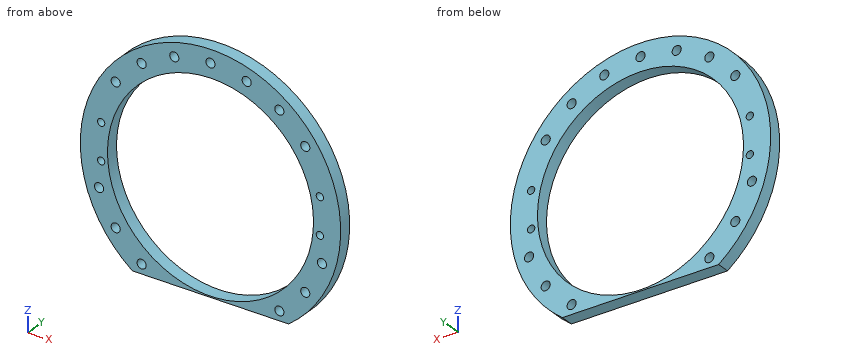
from build123d import *

# Parameters (mm, degrees)
SKETCH4_R           = 50
SKETCH4_R_2         = 39.565
SKETCH4_R_3         = 1.4
SKETCH4_R_4         = 1.75
BOSS_EXTRUDE3_DEPTH = 5
CUT_EXTRUDE1_START  = -40
SKETCH10_W          = 119.00246232
SKETCH10_H          = 31.760523389
CUT_EXTRUDE1_DEPTH  = 31.887234394


with BuildPart() as part:
    # Sketch4 → Boss-Extrude3 (new body)
    with BuildSketch(Plane(origin=(0, 0, 0), x_dir=(1, 0, 0), z_dir=(0, 1, 0))):
        with Locations(Location((0, 0, 0), (0, 0, 270))):
            Circle(SKETCH4_R)
        with Locations(Location((0, 0, 0), (0, 0, 270))):
            Circle(SKETCH4_R_2, mode=Mode.SUBTRACT)
        with Locations(Location((42, -10, 0), (0, 0, 270))):
            Circle(SKETCH4_R_3, mode=Mode.SUBTRACT)
        with Locations(Location((42, 4, 0), (0, 0, 270))):
            Circle(SKETCH4_R_3, mode=Mode.SUBTRACT)
        with Locations(Location((-42, -10, 0), (0, 0, 270))):
            Circle(SKETCH4_R_3, mode=Mode.SUBTRACT)
        with Locations(Location((-42, 4, 0), (0, 0, 270))):
            Circle(SKETCH4_R_3, mode=Mode.SUBTRACT)
        with Locations(Location((0, -45, 0), (0, 0, 270))):
            Circle(SKETCH4_R_4, mode=Mode.SUBTRACT)
        with Locations(Location((-13.905764747, -42.797543233, 0), (0, 0, 270))):
            Circle(SKETCH4_R_4, mode=Mode.SUBTRACT)
        with Locations(Location((-26.450336353, -36.405764747, 0), (0, 0, 270))):
            Circle(SKETCH4_R_4, mode=Mode.SUBTRACT)
        with Locations(Location((-36.405764747, -26.450336353, 0), (0, 0, 270))):
            Circle(SKETCH4_R_4, mode=Mode.SUBTRACT)
        with Locations(Location((-42.797543233, 13.905764747, 0), (0, 0, 270))):
            Circle(SKETCH4_R_4, mode=Mode.SUBTRACT)
        with Locations(Location((-36.405764747, 26.450336353, 0), (0, 0, 270))):
            Circle(SKETCH4_R_4, mode=Mode.SUBTRACT)
        with Locations(Location((-26.450336353, 36.405764747, 0), (0, 0, 270))):
            Circle(SKETCH4_R_4, mode=Mode.SUBTRACT)
        with Locations(Location((26.450336353, 36.405764747, 0), (0, 0, 270))):
            Circle(SKETCH4_R_4, mode=Mode.SUBTRACT)
        with Locations(Location((36.405764747, 26.450336353, 0), (0, 0, 270))):
            Circle(SKETCH4_R_4, mode=Mode.SUBTRACT)
        with Locations(Location((42.797543233, 13.905764747, 0), (0, 0, 270))):
            Circle(SKETCH4_R_4, mode=Mode.SUBTRACT)
        with Locations(Location((36.405764747, -26.450336353, 0), (0, 0, 270))):
            Circle(SKETCH4_R_4, mode=Mode.SUBTRACT)
        with Locations(Location((26.450336353, -36.405764747, 0), (0, 0, 270))):
            Circle(SKETCH4_R_4, mode=Mode.SUBTRACT)
        with Locations(Location((13.905764747, -42.797543233, 0), (0, 0, 270))):
            Circle(SKETCH4_R_4, mode=Mode.SUBTRACT)
    extrude(amount=BOSS_EXTRUDE3_DEPTH)

    # Sketch10 → Cut-Extrude1 (cut, through all)
    with BuildSketch(Plane.XY.offset(CUT_EXTRUDE1_START)):
        with Locations((0.119400464, 6.241721298)):
            Rectangle(SKETCH10_W, SKETCH10_H)
    extrude(amount=-CUT_EXTRUDE1_DEPTH, mode=Mode.SUBTRACT)


solid = part.part
Can you work these out from the model? Positions are in its coordinate system, mm. Coordinates: 2 decimals unless noted, no trailing zeros. Write each loop counter-clockwise with the first axis right and the second up, starting at its lowest first coordinate (ties: lowest second). Pieces come first, ordered by that corner, then holes. Notation, with made-up numbers: (70, -14.75) -> (124, -14.75) arc R20 cw to (124, 11.25) -> close; hole circle Ø4 at (25, -10). An arc over 180 degrees is marked (long way). Write each question's results on one line, items separated by ' | '. Start each with the question number.
Item 1: If we section it at D-D, the plane y = 2.05: Count the separate pieces of the cut face and the enclosed holes in it, and give its area (3 significant figures).
Item 2: If we section it at B-B, the plane x = 0: Write out the boundary of the cut face in (y, z) (3 decimals).
Item 3: I'm going to push flat-ended pins straight in: P1, Ø1.5, axis at y = 3, z = -8, coming from the +X side; P2, Ø1, axis at x = 1, y = 2, coming from the +Z side; P3, Ø4, axis at x = 13.91, z = 42.8, coming from the -Y side. Where does each tip first touch, or does it pass through?
Item 4: Please list where these lines run through material, in increasing order: probe 1 along X at (y, z) = (3.75, 10); probe 2 along Z at (x, y) = (-35, 0.7); probe 3 along Z at (x, y) = (-1, 3.45).
Item 5: If we section it at A-A, the plane z = 0: Write out the boundary of the cut face in (x, y) (3 decimals), and give its area (3 significant figures).
Item 6: If we section it at C-C, the plane z = 10: Write out the boundary of the cut face in (x, y), and give its area (3 significant figures).
Answer block:
1) separate pieces: 1 | enclosed holes: 18 | area: 2,380 mm²
2) outline: (0, -40) -> (5, -40) -> (5, -39.565) -> (0, -39.565) -> close; (0, 39.565) -> (5, 39.565) -> (5, 43.25) -> (0, 43.25) -> close; (0, 46.75) -> (5, 46.75) -> (5, 50) -> (0, 50) -> close
3) P1: x = 49.47 | P2: z = 50 | P3: y = 0
4) probe 1: -48.99 to -43.4, -40.6 to -38.28, 38.28 to 40.6, 43.4 to 48.99 | probe 2: -35.71 to -27.49, -25.41 to -18.45, 18.45 to 25.41, 27.49 to 35.71 | probe 3: -40 to -39.55, 39.55 to 43.56, 46.44 to 49.99
5) outline: (-50, 0) -> (-39.565, 0) -> (-39.565, 5) -> (-50, 5) -> close; (39.565, 0) -> (50, 0) -> (50, 5) -> (39.565, 5) -> close | area: 104 mm²
6) outline: (-48.99, 0) -> (-43.4, 0) -> (-43.4, 5) -> (-48.99, 5) -> close; (-40.6, 0) -> (-38.28, 0) -> (-38.28, 5) -> (-40.6, 5) -> close; (38.28, 0) -> (40.6, 0) -> (40.6, 5) -> (38.28, 5) -> close; (43.4, 0) -> (48.99, 0) -> (48.99, 5) -> (43.4, 5) -> close | area: 79.1 mm²
